```python
from build123d import *

# Parameters (mm, degrees)
CROQUIS2_R                = 4.7625
SALIENTE_EXTRUIR1_DEPTH   = 24.384
CHAFL_N1_SIZE             = 0.396875
CLEARANCE_HOLE_DEPTH      = 26.297080237
CLEARANCE_HOLE_DEPTH_BACK = 26.297080237
CROQUIS4_R                = 2.4892


with BuildPart() as part:
    # Croquis2 → Saliente-Extruir1 (new, symmetric)
    with BuildSketch(Plane(origin=(0, 0, 0), x_dir=(1, 0, 0), z_dir=(0, 1, 0))):
        with Locations(Location((0, 0, 0), (0, 0, 90))):
            Circle(CROQUIS2_R)
    extrude(amount=SALIENTE_EXTRUIR1_DEPTH, both=True)

    # Chafl_n1
    chafl_n1_edges = [part.edges().sort_by_distance(p)[0] for p in [
        (0, -24.384, 4.7625),
        (0, 24.384, 4.7625),
    ]]
    chamfer(chafl_n1_edges, length=CHAFL_N1_SIZE)

    # Croquis4 → Clearance Hole (cut, two sides: drawn at the far end of the back side and taken through both)
    with BuildSketch(Plane(origin=(0, 0, 0), x_dir=(1, 0, 0), z_dir=(0, 1, 0)).offset(-CLEARANCE_HOLE_DEPTH_BACK)):
        with Locations(Location((0, 0, 0), (0, 0, 270))):
            Circle(CROQUIS4_R)
    extrude(amount=CLEARANCE_HOLE_DEPTH + CLEARANCE_HOLE_DEPTH_BACK, mode=Mode.SUBTRACT)


solid = part.part
```
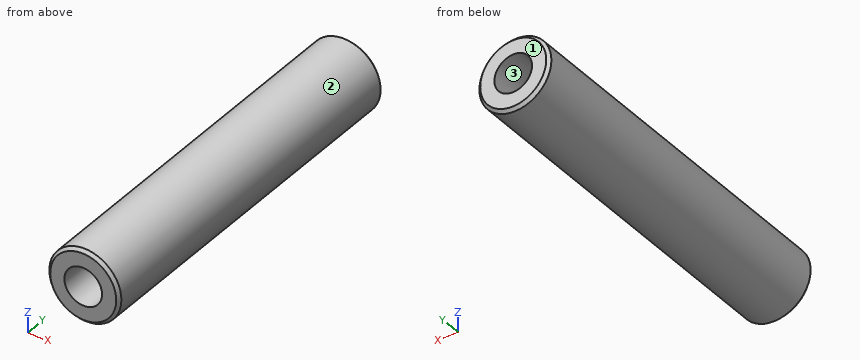
Build history of the part. All positions in model axes, mm. Face numbers are marked on the shaded views. Give positions to 0.01 mm unless a question says otherwise; leave off trailing zeros. Loops run counter-clockwise (first coordinate to the right, second up) from the corner with the lowest first, then second, coordinate; pieces in that order, holes last.
Item 1: Flat gauge pins, fed straight in: pin 1 (1 mm diameter, centred on x = -2, y = 14.5, fed in from +Z); pin 2 (1 mm diameter, centred on y = 5.5, z = 0.5, fed in from +X); pin 3 (3 mm diameter, centred on x = -2, y = -18.5, fed in from +Z); pin 4 (2 mm diameter, centred on y = 13, z = 3, fed in from -X). Where does each tip first touch, or does it go through?
Answers follow:
pin 1: stops at z = 4.52
pin 2: stops at x = 4.76
pin 3: stops at z = 4.74
pin 4: stops at x = -4.32
Item 2: Drill centre lines: line 1 (X direction, y = 14, z = 0); line 2 (Z direction, x = 1, y = 19); line 3 (Z direction, x = 0.5, y = 15.5). Where is each one in solid material? Low to high.
Answers follow:
line 1: x = -4.76 to -2.49, 2.49 to 4.76
line 2: z = -4.66 to -2.28, 2.28 to 4.66
line 3: z = -4.74 to -2.44, 2.44 to 4.74
Item 3: Slice it at B-B, the plane z = 0. List the corners of the cut face in (x, y).
Answers follow:
outline: (-4.76, -23.99) - (-4.37, -24.38) - (-2.49, -24.38) - (-2.49, 24.38) - (-4.37, 24.38) - (-4.76, 23.99) - close; (2.49, -24.38) - (4.37, -24.38) - (4.76, -23.99) - (4.76, 23.99) - (4.37, 24.38) - (2.49, 24.38) - close
Item 4: Slice it at A-A, the plane x = 0. List the corners of the cut face in (y, z).
Answers follow:
outline: (-24.38, -4.37) - (-23.99, -4.76) - (23.99, -4.76) - (24.38, -4.37) - (24.38, -2.49) - (-24.38, -2.49) - close; (-24.38, 2.49) - (24.38, 2.49) - (24.38, 4.37) - (23.99, 4.76) - (-23.99, 4.76) - (-24.38, 4.37) - close
Item 5: Pull direction X, two halves, no side cores. Call the marked faces 1, 2 and 3: released by +X, released by -X, zero draft, split by the parting line, or undercut.
Answers follow:
face 1: zero draft
face 2: split by the parting line
face 3: undercut
Item 6: Slice it at C-C, the plane y = 0. List the corners of the cut face in (x, z) (1 decimal).
Answers follow:
outline: circle Ø9.5 at (0, 0); hole circle Ø5 at (0, 0)
